Geometry: final body of the model. Coordinates: model frame, mm. Round coordinates to 2 decimals unless told otherwise and drop trailing zeros. Loops run counter-clockwise (first coordinate to the right, second up) from the corner with the lowest first, then second, coordinate; pieces in that order, holes last. Notation, with made-up numbers: (73.25, 27) -> (121.25, 27) arc R20 ccw to (121.25, 37) -> close; hole circle Ø11 at (28.25, 86.5). An arc over 180 degrees is marked (long way). Answer in a Markdown table with one row per item.
```python
from build123d import *

# Parameters (mm, degrees)
F1_R = 19.05
F5_R = 19.05


with BuildPart() as f2:
    # F2: sweep along a path in F0
    with BuildLine(Plane.XY) as f2_path:
        Line((-267.4559177475, 641.6957181156), (265.9440822525, 641.6957181156))
        ThreePointArc((265.9440822525, 641.6957181156), (292.8848506157, 630.5364864788), (304.0440822525, 603.5957181156))
        Line((304.0440822525, 603.5957181156), (304.0440822525, -539.4042818844))
        ThreePointArc((304.0440822525, -539.4042818844), (292.8848506157, -566.3450502476), (265.9440822525, -577.5042818844))
        Line((265.9440822525, -577.5042818844), (-267.4559177475, -577.5042818844))
        ThreePointArc((-267.4559177475, -577.5042818844), (-294.3966861107, -566.3450502476), (-305.5559177475, -539.4042818844))
        Line((-305.5559177475, -539.4042818844), (-305.5559177475, 603.5957181156))
        ThreePointArc((-305.5559177475, 603.5957181156), (-294.3966861107, 630.5364864788), (-267.4559177475, 641.6957181156))
    # F1 (on Right) → F2 (sweep)
    with BuildSketch(Plane.YZ):
        with Locations((641.6957181156, 0)):
            Circle(F1_R)
    sweep(path=f2_path.line)

    # F6: sweep along a path in F4
    with BuildLine(Plane.YZ.offset(254)) as f6_path:
        Line((641.6957181156, 0), (426.7178632358, 1219.2))
        Line((426.7178632358, 1219.2), (-362.5264270047, 1219.2))
        Line((-362.5264270047, 1219.2), (-577.5042818844, 0))
    # F5 (on Front) → F6 (sweep)
    with BuildSketch(Plane.XZ):
        with Locations((254, 1219.2)):
            Circle(F5_R)
    sweep(path=f6_path.line, transition=Transition.RIGHT)


solid = f2.part
```
Item 1: First-contact query: P1, Ø1, axis at x = 254.5, z = 521.5, coming from the +Y side. Flat tip, straight axial feed; report the tip coordinate or a pass-through.
Ans:
| item | result |
|---|---|
| P1 | y = 569.17 |
Item 2: Ray query, L1, parallel to Y at x = 265.5, z = 385; L2, parallel to Y at x = 269.5, z = 387.5; L3, parallel to X at y = -460.5, z = 755. Return the intervals inside material, ascending.
Ans:
| item | result |
|---|---|
| L1 | -525.04 to -494.2, 558.39 to 589.23 |
| L2 | -520.42 to -497.93, 562.12 to 584.61 |
| L3 | 243.47 to 264.53 |
Item 3: Section query C-C, the plane y = 521. State how many separate pieces and enclosed holes the cut face has, and give its area (3 significant figures).
Ans:
| item | result |
|---|---|
| separate pieces | 3 |
| enclosed holes | 0 |
| area | 8,850 mm2 |
Item 4: Section query B-B, the plane y = 88.5. Output: boundary loops of the cut face in (x, z), and give its area (3 significant figures).
Ans:
| item | result |
|---|---|
| outline | circle Ø38.1 at (-305.56, 0); circle Ø38.1 at (254, 1219.2); circle Ø38.1 at (304.04, 0) |
| area | 3,420 mm2 |
Item 5: Section query A-A, the plane x = -127. Output: boundary loops of the cut face in (y, z).
Ans:
| item | result |
|---|---|
| outline | circle Ø38.1 at (-577.5, 0); circle Ø38.1 at (641.7, 0) |
